The figure shows three views and two pictorial views of one solid part (mm, origin at its lowest corner). Answer the questions. Give positions to 0.01 mm unless a question says otherwise; leave off trailing zeros. Order: outer loops, then holes, each group sorted by start corner. A loop starts at its lowest first (then second) coordinate and runs counter-clockwise, first axis right, second up. Notation, with made-up numbers: M 23.25,62 L 28.25,62 A21 ccw 28.25,90 Z; hole C 65,72 d3. An arc over 180 degrees is marked long. Write item = value, one per line. Start each with the question number.
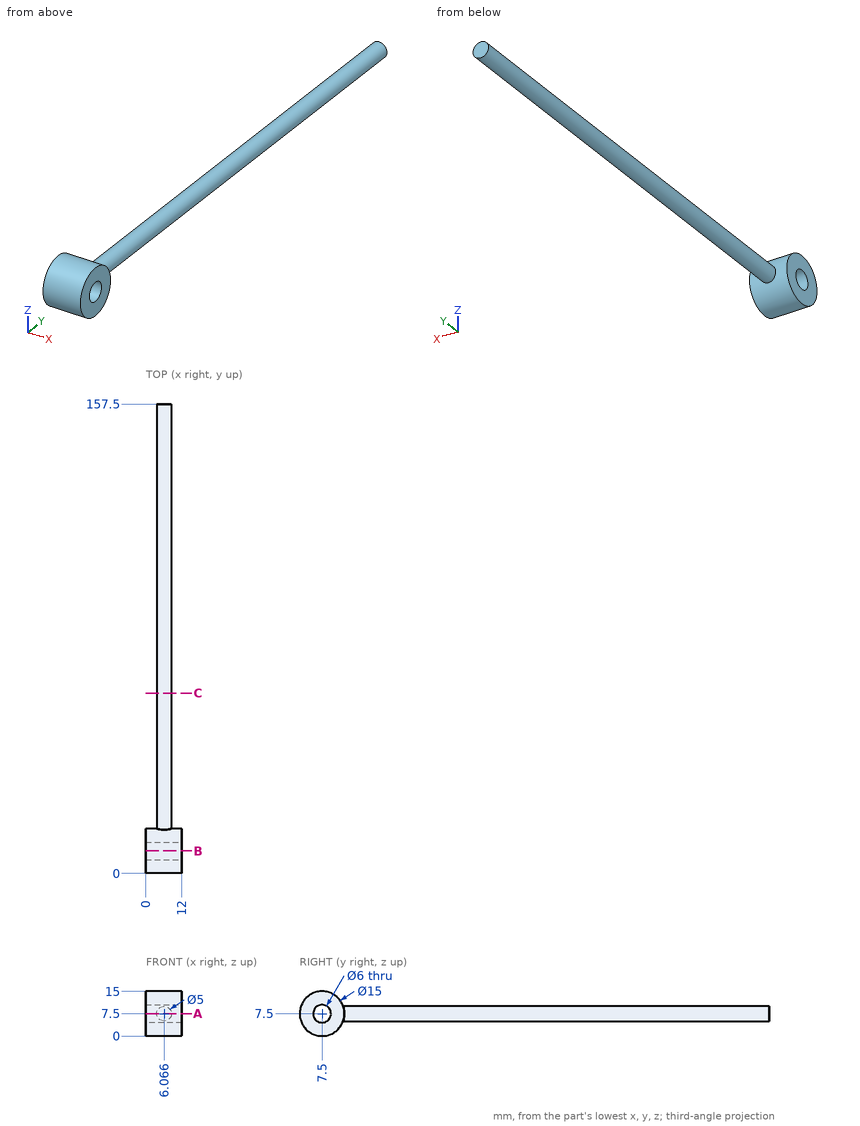
1) Find the intervals of material crossed by probe 1 along Y at (x, z) = (3.75, 7.75) (1 decimal); probe 2 along Y at (x, z) = (3, 7.5); probe 3 along Z at (x, y) = (4.75, 88.5) (1 decimal), in increasing order. Write a range as [from, to].
2) Find section A-A on z = 7.5. Determine the outline of the cut face in (x, y) (1 decimal).
3) Find section B-B on y = 7.5. Determine the outline of the cut face in (x, z).
4) Find section C-C on y = 60.5. Determine the outline of the cut face in (x, z) (1 decimal).
5) Each of these flat-tipped pins is pushed along its axis until it touches: P1, Ø3, axis at x = 9, z = 5, coming from the -Y side; P2, Ø1.5, axis at y = 109, z = 11.5, coming from the +X side; P3, Ø2, axis at x = 2.5, z = 12.5, coming from the -Y side (1 decimal); P4, Ø8, axis at y = 85, z = 11, coming from the +X side. Where does it stop, or does it pass through?
Numbers:
q1.probe_1 = [0, 4.5], [10.5, 157.5]
q1.probe_2 = [0, 4.5], [10.5, 15]
q1.probe_3 = [5.4, 9.6]
q2.outline = M 0,0 L 12,0 L 12,4.5 L 0,4.5 Z; M 0,10.5 L 12,10.5 L 12,15 L 8.6,15 L 8.6,157.5 L 3.6,157.5 L 3.6,15 L 0,15 Z
q3.outline = M 0,0 L 12,0 L 12,4.5 L 0,4.5 Z; M 0,10.5 L 12,10.5 L 12,15 L 0,15 Z
q4.outline = C 6.1,7.5 d5
q5.P1 = 0.07
q5.P2 = through
q5.P3 = 1.2
q5.P4 = 8.57
